Geometry check sheet. Reference: the model listing, model coordinates, mm. Give positions to 0.01 mm unless a question says otherwise; leave off trailing zeros. Write each loop counter-clockwise with the first axis right and the second up, starting at its lowest first coordinate (ties: lowest second). Pieces come first, ordered by that corner, then holes. Notation, with made-up numbers: (89, 14.5) - (119, 14.5) arc R25 cw to (119, 52.5) - close; hole circle Ø1 at (-15.75, 63). An arc over 180 degrees is marked (long way). One line per question, with ' | ' between items. Start each with the question number.
Q1. Section check C-C on z = -6.5. Record the boundary of the cut face in (x, y), and give its area (3 significant figures).
Q2. Gauge pin test, flat ends, axial feed: P1, Ø2, axis at x = 22.5, y = 1.5, coming from the -Z side; P2, Ø3, axis at x = -16, z = -5, coming from the -Y side; P3, Ø2, axis at x = -4.5, y = 1, coming from the +Z side; P4, Ø4, axis at x = 13, z = -4.5, coming from the -Y side. Record the tip position at first contact, or that the pin passes through.
Q3. Section check A-A on z = 8. Record the boundary of the cut face in (x, y).
Q4. Section check B-B on y = -0.5. Record the boundary of the cut face in (x, z), and give its area (3 significant figures).
Q5. Section check D-D on x = 4.5. Record the boundary of the cut face in (y, z), and give its area (3 significant figures).
Q6. Thickness scan on L1, parallel to Z at x = 5, y = 0.3; L2, parallel to X at y = -1.7, z = 5.75; L3, parallel to X at y = 1.55, z = -7.5. Record the ranges inside material, lowest first. Write a range as [from, to].
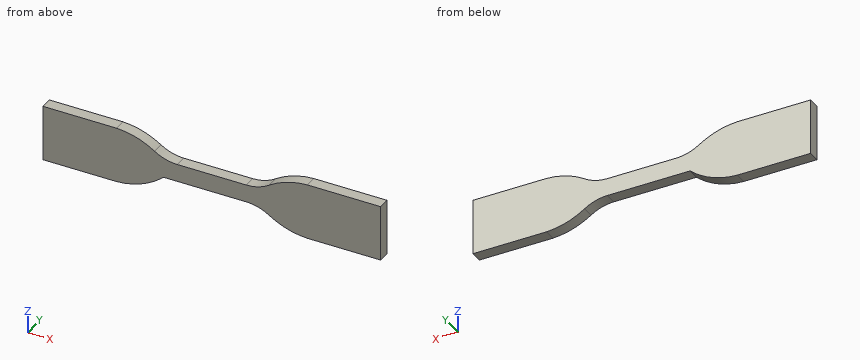
```python
from build123d import *

# Parameters (mm, degrees)
F1_DEPTH = 2


with BuildPart() as f1:
    # F0 (on Front) → F1 (new body, symmetric)
    with BuildSketch(Plane.XZ):
        with BuildLine():
            Line((11.751494, 3), (0, 3))
            Line((0, 3), (-11.751494, 3))
            ThreePointArc((-11.751494, 3), (-15.797231, 3.597313), (-19.497744, 5.338285))
            ThreePointArc((-19.497744, 5.338285), (-25.709291, 8.323868), (-32.5, 9.5))
            Line((-32.5, 9.5), (-57.5, 9.5))
            Line((-57.5, 9.5), (-57.5, 0))
            Line((-57.5, 0), (-57.5, -9.5))
            Line((-57.5, -9.5), (-32.5, -9.5))
            ThreePointArc((-32.5, -9.5), (-25.709291, -8.323868), (-19.497744, -5.338285))
            ThreePointArc((-19.497744, -5.338285), (-17.954359, -4.22621), (-16.5, -3))
            Line((-16.5, -3), (-11.751494, -3))
            Line((-11.751494, -3), (0, -3))
            Line((0, -3), (11.751494, -3))
            ThreePointArc((11.751494, -3), (15.797231, -3.597313), (19.497744, -5.338285))
            ThreePointArc((19.497744, -5.338285), (25.709291, -8.323868), (32.5, -9.5))
            Line((32.5, -9.5), (57.5, -9.5))
            Line((57.5, -9.5), (57.5, 0))
            Line((57.5, 0), (57.5, 9.5))
            Line((57.5, 9.5), (32.5, 9.5))
            ThreePointArc((32.5, 9.5), (25.709291, 8.323868), (19.497744, 5.338285))
            ThreePointArc((19.497744, 5.338285), (15.797231, 3.597313), (11.751494, 3))
        make_face()
    extrude(amount=F1_DEPTH, both=True)


solid = f1.part
```
Working result:
1) outline: (-57.5, -2) - (-21.43, -2) - (-21.43, 2) - (-57.5, 2) - close; (21.43, -2) - (57.5, -2) - (57.5, 2) - (21.43, 2) - close | area: 289 mm2
2) P1: stops at z = -7.5 | P2: passes through | P3: stops at z = 3 | P4: stops at y = -2
3) outline: (-57.5, -2) - (-24.76, -2) - (-24.76, 2) - (-57.5, 2) - close; (24.76, -2) - (57.5, -2) - (57.5, 2) - (24.76, 2) - close
4) outline: (-57.5, -9.5) - (-32.5, -9.5) arc R25 ccw to (-19.5, -5.34) arc R25 ccw to (-16.5, -3) - (11.75, -3) arc R14 cw to (19.5, -5.34) arc R25 ccw to (32.5, -9.5) - (57.5, -9.5) - (57.5, 9.5) - (32.5, 9.5) arc R25 ccw to (19.5, 5.34) arc R14 cw to (11.75, 3) - (-11.75, 3) arc R14 cw to (-19.5, 5.34) arc R25 ccw to (-32.5, 9.5) - (-57.5, 9.5) - close | area: 1,630 mm2
5) outline: (-2, -3) - (2, -3) - (2, 3) - (-2, 3) - close | area: 24.0 mm2
6) L1: z = [-3, 3] | L2: x = [-57.5, -20.14], [20.14, 57.5] | L3: x = [-57.5, -23.5], [23.5, 57.5]
